Geometry check sheet. Reference: the model listing, model coordinates, mm. Face numbers are marked on the shaded views. Round coordinates to 2 decimals unless told otherwise and drop trailing zeros. Order: outer loops, then holes, each group sorted by start corner. A loop starts at its lowest first (then second) coordinate and runs counter-clockwise, first axis right, second up.
Autodesk Inventor part; units mm, degrees
ref_plane "YZ Plane" through (0, 0, 0) normal (1, 0, 0) x (0, 1, 0)
ref_plane "XZ Plane" through (0, 0, 0) normal (0, 1, 0) x (-1, 0, 0)
ref_plane "XY Plane" through (0, 0, 0) normal (0, 0, 1) x (1, 0, 0)
sketch "Skizze1" plane through (0, 0, 0) normal (0, 1, 0) x (-1, 0, 0)
  circle A0 centre (0, 0) radius 28
  circle A1 centre (0, 0) radius 30
  dimension "d0" = 56
  dimension "d1" = 60
extrude "Extrusion1" add sketch "Skizze1" along normal mid plane 10
sketch "Skizze2" plane through (0, 0, 0) normal (0, 1, 0) x (-1, 0, 0)
  circle A0 centre (0, 22.5) radius 4.25
  circle A1 centre (0, -22.5) radius 4.25
  line L0 (44.9262, 0) -> (-43.1306, 0) construction
  circle A2 centre (0, -22.5) radius 6.5
  circle A3 centre (0, 22.5) radius 6.5
  line L1 (0, 38.6377) -> (0, -60.2779) construction
  line L2 (3, 29.5) -> (-3, 29.5)
  line L3 (-3, 29.5) -> (-3, -29.5)
  line L4 (-3, -29.5) -> (3, -29.5)
  line L5 (3, -29.5) -> (3, 29.5)
  point P0 (0, 0)
  point P1 (-3, 28.2663)
  point P2 (3, 28.2663)
  point P3 (-3, -28.2663)
  point P4 (3, -28.2663)
  dimension "d4" = 45
  dimension "d5" = 8.5
  dimension "d6" = 8.5
  dimension "d7" = 13
  dimension "d8" = 13
  dimension "d9" = 6
  dimension "d21" = 59
extrude "Extrusion2" add sketch "Skizze2" along normal mid plane 5 contours A0 L5 A3 | A0 L3 A3 L5 | L5 A3 L3 A0 | A0 L3 A3 | A3 L3 L2 L5 | L5 A1 L3 A2 | A2 L5 A1 | L3 A1 A2 | L3 A1 L5 A2 | A2 L5 L4 L3
sketch "Skizze3" plane through (0, 0, 0) normal (0, 1, 0) x (-1, 0, 0)
  line L0 (-37.328, 53.3099) -> (47.5678, -67.9338) construction
  line L1 (48.5469, 69.3321) -> (-29.5635, -42.2211) construction
  line L2 (0, 56.0595) -> (0, -79.5026) construction
  circle A0 centre (0, 0) radius 30
  circle A1 centre (0, 0) radius 28
  line L3 (19.8236, 28.311) -> (13.732, 19.6114)
  line L4 (14.4871, -20.6897) -> (22.3283, -31.8882)
  point P0 (16.0601, -22.9363)
  point P1 (17.2073, -24.5746)
  point P2 (17.2073, 24.5746)
  point P3 (16.0601, 22.9363)
  dimension "d12" = 110
  dimension "d13" = 35
  dimension "d19" = 56
  dimension "d20" = 60
extrude "Extrusion3" cut sketch "Skizze3" along normal mid plane 10 contours A0 L4 A1 L3 picked at (29.0468, 2.3769)
fillet "Rundung1" radius 4 4 edges at (-16.6337, -5, -23.7554) (-16.6337, 5, -23.7554) (-16.6337, 5, 23.7554) (-16.6337, -5, 23.7554)
fillet "Rundung2" radius 2 4 edges at (3.8552, 0, -27.7333) (-3.8552, 0, -27.7333) (-3.8552, 0, 27.7333) (3.8552, 0, 27.7333)
properties part number "_3D-Druck"
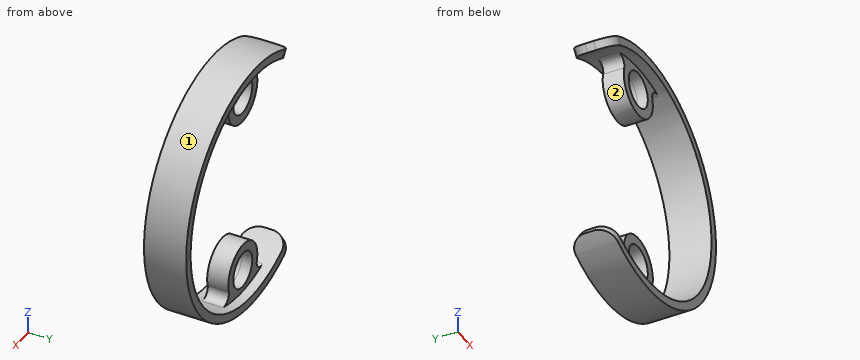
(1) Sectioned sample at D-D, the plane y = -1.75. Give the number of separate pieces and of enclosed holes in the cut face, and give its area (3 significant figures).
Returned:
separate pieces: 1
enclosed holes: 2
area: 411 mm2
(2) Sectioned sample at B-B, the plane x = 22. Record the cut outline in (y, z).
Returned:
outline: (-5, -20.4) - (5, -20.4) - (5, -17.32) - (-5, -17.32) - close; (-5, 17.32) - (5, 17.32) - (5, 20.4) - (-5, 20.4) - close
(3) Sectioned sample at A-A, the plane x = 0. Record the cut outline in (y, z), and give its area (3 significant figures).
Returned:
outline: (-5, -30) - (5, -30) - (5, -28) - (2.5, -28) - (2.5, -26.75) - (-2.5, -26.75) - (-2.5, -28) - (-5, -28) - close; (-5, 28) - (-2.5, 28) - (-2.5, 26.75) - (2.5, 26.75) - (2.5, 28) - (5, 28) - (5, 30) - (-5, 30) - close; (-2.5, -18.25) - (2.5, -18.25) - (2.5, -16) - (-2.5, -16) - close; (-2.5, 16) - (2.5, 16) - (2.5, 18.25) - (-2.5, 18.25) - close
area: 75.0 mm2
(4) Sectioned sample at C-C, the plane z = 0. Record the cut outline in (x, y).
Returned:
outline: (28, -5) - (30, -5) - (30, 5) - (28, 5) - close
(5) Draft check along Z on the marked faces 1 and 2. Enter one of: released by +Z, released by -Z, zero draft, split by the parting line, or undercut.
Returned:
face 1: split by the parting line
face 2: undercut
(6) Depth check by flat-ended pin: P1, Ø13, axis at x = -0.5, z = 20, coming from the -Y side; P2, Ø2, axis at y = 0.5, z = -6, coming from the -X side; P3, Ø4, axis at y = -4, z = -19.5, coming from the +X side. Enter the tip coordinate at first touch or a pass-through.
Returned:
P1: stops at y = -2.5
P2: stops at x = 27.11
P3: stops at x = 24.37
(7) Material ranges on line 1 (Z direction, x = 0, y = 1.65); line 2 (X direction, y = -1.5, z = -22.5); line 3 (Z direction, x = 1.5, y = 0), recorded low to high.
Returned:
line 1: z = -30 to -26.75, -18.25 to -16, 16 to 18.25, 26.75 to 30
line 2: x = -6.5 to -4.25, 4.25 to 6.5, 16.67 to 19.84
line 3: z = -29.96 to -26.48, -18.52 to -16.18, 16.18 to 18.52, 26.48 to 29.96
